Read the model definition and answer for the solid it produces. Units are mm, in the model's axes. A direction names the side the tool comes from. Coordinates: 2 decimals unless noted, no trailing zeros. Write each loop counter-clockwise with the first axis right and the second up, starting at its lowest first coordinate (ties: lowest second). Pieces come first, ordered by that corner, then holes. Notation, with made-up numbers: (50.25, 33.5) -> (86.25, 33.5) arc R4 cw to (86.25, 39.5) -> close; hole circle Ø2 at (63, 72). An arc over 180 degrees is marked (long way). Answer in a Markdown table with one row per item. Add a question column.
Item 1: Section A-A on y = -7.25 is taken. Write down the section's boundary in (x, z).
Item 2: Which of the six approach directions +Z, -Z, +X, -X, +Y, -Y give full straight-line access (tool end or side, diameter ignored) to faces 1 (the face through (-5, 8.3, -8.89)), 2 (the face through (10.6, 3.34, -4.38)), 3 (the face through (5, -5, 0))?
Item 3: Given pin 1 Ø8 at (y, z) = (5, 2) entering from +X; pin 2 Ø6 at (y, z) = (-6.5, -7.5) entering from -X; pin 3 Ø1 at (x, z) = (4.5, 2) entering from +Y, each flat-ended and moving along its own axis, determine where each tip first touches the part or whether it passes through.
Item 4: Section D-D on y = 5.5 is taken. Write down the section's boundary in (x, z) (3 decimals).
Item 5: Straight lines are drawn through the part: line 1 (Z direction, x = -9.25, y = -4.25); line 2 (Z direction, x = 2.5, y = 6.75); line 3 (X direction, y = 0, z = -11.5) (3 decimals). For each, find the intervals that lie inside material, in ascending order. Write a range as from..to.
Item 6: Section C-C on z = -13.25 is taken. Write down the section's boundary in (x, y) (3 decimals).
```python
from build123d import *

# Parameters (mm, degrees)
SKETCH1_R      = 6.35
EXTRUDE1_DEPTH = 9.525
SKETCH2_R      = 9.525
EXTRUDE2_DEPTH = 19.05
SKETCH3_R      = 11.1125
EXTRUDE3_DEPTH = 8.89


with BuildPart() as part:
    # Sketch1 → Extrude1 (new body)
    with BuildSketch(Plane.XY):
        Circle(SKETCH1_R)
    extrude(amount=EXTRUDE1_DEPTH)

    # Sketch2 → Extrude2 (add)
    with BuildSketch(Plane(origin=(0, 0, 0), x_dir=(-1, 0, 0), z_dir=(0, 0, -1))):
        Circle(SKETCH2_R)
    extrude(amount=EXTRUDE2_DEPTH)

    # Sketch3 → Extrude3 (add)
    with BuildSketch(Plane.XY):
        Circle(SKETCH3_R)
    extrude(amount=-EXTRUDE3_DEPTH)


solid = part.part
```
Results below:
| question | item | result |
|---|---|---|
| 1 | outline | (-8.42, -8.89) -> (-6.18, -8.89) -> (-6.18, -19.05) -> (6.18, -19.05) -> (6.18, -8.89) -> (8.42, -8.89) -> (8.42, 0) -> (-8.42, 0) -> close |
| 2 | face 1 | -Z |
| 2 | face 2 | +Z, -Z |
| 2 | face 3 | +Z |
| 3 | pin 1 | stops at x = 11.01 |
| 3 | pin 2 | stops at x = -10.55 |
| 3 | pin 3 | stops at y = 4.93 |
| 4 | outline | (-9.656, -8.89) -> (-7.777, -8.89) -> (-7.777, -19.05) -> (7.777, -19.05) -> (7.777, -8.89) -> (9.656, -8.89) -> (9.656, 0) -> (3.174, 0) -> (3.174, 9.525) -> (-3.174, 9.525) -> (-3.174, 0) -> (-9.656, 0) -> close |
| 5 | line 1 | z = -8.89..0 |
| 5 | line 2 | z = -19.05..0 |
| 5 | line 3 | x = -9.525..9.525 |
| 6 | outline | circle Ø19.05 at (0, 0) |
